```python
from build123d import *

# Parameters (mm, degrees)
PAD_DEPTH       = 49.15
POCKET_DEPTH    = 3.2
CHAMFER_SIZE    = 0.5
POCKET001_DEPTH = 45.001


with BuildPart() as body:
    # Sketch → Pad (new body)
    with BuildSketch(Plane.XZ):
        Polygon((25.980762, 0), (12.990381, 22.5), (-12.990381, 22.5), (-25.980762, 0), (-12.990381, -22.5), (12.990381, -22.5), align=None)
    extrude(amount=PAD_DEPTH)

    # Sketch017 → Pocket (cut)
    with BuildSketch(Plane(origin=(0, 0, 0), x_dir=(1, 0, 0), z_dir=(0, 1, 0))):
        Polygon((17.205038, 0), (8.602519, 14.9), (-8.602519, 14.9), (-17.205038, 0), (-8.602519, -14.9), (8.602519, -14.9), align=None)
    extrude(amount=-POCKET_DEPTH, mode=Mode.SUBTRACT)

    # Chamfer
    chamfer_edges = [body.edges().sort_by_distance(p)[0] for p in [
        (12.903779, 0, 7.45),
        (12.903779, 0, -7.45),
        (0, 0, -14.9),
        (-12.903779, 0, -7.45),
        (-12.903779, 0, 7.45),
        (0, 0, 14.9),
    ]]
    chamfer(chamfer_edges, length=CHAMFER_SIZE)

    # Sketch018 (on Face10 of Chamfer) → Pocket001 (cut, through all)
    with BuildSketch(Plane(origin=(0, 0, 22.5), x_dir=(-1, 0, 0), z_dir=(0, 0, 1))):
        with BuildLine():
            ThreePointArc((-9.5, 16), (0, 6.5), (9.5, 16))
            Line((9.5, 49.15), (9.5, 16))
            Line((-9.5, 49.15), (9.5, 49.15))
            Line((-9.5, 16), (-9.5, 49.15))
        make_face()
    extrude(amount=-POCKET001_DEPTH, mode=Mode.SUBTRACT)


with BuildPart() as part_mirroring:
    # Part__Mirroring: instance of Body
    add(body.part.mirror(Plane(origin=(0, 0, 0), x_dir=(1, 0, 0), z_dir=(0, 1, 0))))


with BuildPart() as part_mirroring_1:
    # Part__Mirroring placement: moved
    add(part_mirroring.part.moved(Location((0, -98.3, 0))))


solid = part_mirroring_1.part
```
The listing builds one solid part. Answer for the finished solid, in the listing's coordinates (mm). A direction names the side the tool comes from. Give positions to 0.01 mm unless a question says otherwise; leave off trailing zeros. Order: outer loops, then holes, each group sorted by start corner. A loop starts at its lowest first (then second) coordinate and runs counter-clockwise, first axis right, second up. Notation, with made-up numbers: (-27.75, 71.5) - (4.25, 71.5) arc R22 ccw to (4.25, 101.5) - close; hole circle Ø6 at (19, -39.5). An arc over 180 degrees is marked (long way). Use one line per item in the form item = value. Start each with the question number.
(1) A cutting plane is placed at A-A, the plane y = -67. Write down the section's boundary in (x, z).
(2) The mould has two halves that part along Z. Classify faces 4 (the flat face through (10, -81, -22.5)), 5 (the flat face through (12.844, -96.469, 7.554)), 6 (the flat face through (-16, -49.15, 0)): released by +Z, released by -Z, zero draft, split by the parting line, or undercut.
(3) Flat-ended cylindrical pins translate along their axes: pin 1 Ø8 at (x, y) = (-20, -86.5) entering from +Z; pin 2 Ø10 at (y, z) = (-64.5, 7) entering from -X; pin 3 Ø15 at (x, z) = (7.5, 2.5) entering from -Y. Find the tip coordinate at first contact, or state that the pin passes through.
(4) A cutting plane is placed at D-D, the plane y = -93. Write down the section's boundary in (x, z).
(5) Consider line 1 (X direction, y = -67.5, z = 12); line 2 (X direction, y = -72, z = 9.5); line 3 (Y direction, x = 10, z = 8). Determine where each line is inside the solid, lowest interval first. Write a range as from..to.
(6) A cutting plane is placed at C-C, the plane z = -3. Write down the section's boundary in (x, y), then the cut area to 3 significant figures.
(7) For faces 1 (the flat face through (12.96, -96.47, -7.35)), 2 (the flat face through (16, -49.15, 0)), 3 (the flat face through (-9.5, -65, 0)), determine the directions among +Z, -Z, +X, -X, +Y, -Y from which every point of the face is accessible in a straight line to the end or side of a thin tool.
(8) A cutting plane is placed at B-B, the plane x = 0. Write down the section's boundary in (y, z).
Ans:
q1.outline = (-25.98, 0) - (-12.99, -22.5) - (-9.5, -22.5) - (-9.5, 22.5) - (-12.99, 22.5) - close; (9.5, -22.5) - (12.99, -22.5) - (25.98, 0) - (12.99, 22.5) - (9.5, 22.5) - close
q2.face_4 = released by -Z
q2.face_5 = undercut
q2.face_6 = zero draft
q3.pin_1 = 17.29
q3.pin_2 = -24.83
q3.pin_3 = -98.15
q4.outline = (-25.98, 0) - (-12.99, -22.5) - (12.99, -22.5) - (25.98, 0) - (12.99, 22.5) - (-12.99, 22.5) - close
q5.line_1 = -19.05..-9.5, 9.5..19.05
q5.line_2 = -20.5..-9.5, 9.5..20.5
q5.line_3 = -95.1..-49.15
q6.outline = (-24.25, -98.3) - (-16.05, -98.3) - (-15.47, -97.8) - (-15.47, -95.1) - (15.47, -95.1) - (15.47, -97.8) - (16.05, -98.3) - (24.25, -98.3) - (24.25, -49.15) - (9.5, -49.15) - (9.5, -82.3) arc R9.5 cw to (-9.5, -82.3) - (-9.5, -49.15) - (-24.25, -49.15) - close
q6.area = 1,510 mm^2
q7.face_1 = -Y
q7.face_2 = +Z, -Z, +X, -X, +Y
q7.face_3 = +Z, -Z, +Y
q8.outline = (-98.3, -22.5) - (-91.8, -22.5) - (-91.8, 22.5) - (-98.3, 22.5) - (-98.3, 15.4) - (-97.8, 14.9) - (-95.1, 14.9) - (-95.1, -14.9) - (-97.8, -14.9) - (-98.3, -15.4) - close
